```python
from build123d import *

# Parameters (mm, degrees)
SKETCH1_W             = 40
SKETCH1_H             = 84
SKETCH1_R             = 10.5
BOSS_EXTRUDE1_DEPTH   = 6
SKETCH2_W             = 40
SKETCH2_H             = 32
BOSS_EXTRUDE2_DEPTH   = 13
F_6_0MM_DOWEL_HOLE1_D = 6
M5_CLEARANCE_HOLE1_D  = 5.5
M4X0_7_TAPPED_HOLE1_D = 3.3
SKETCH12_R            = 17.5
CUT_EXTRUDE1_DEPTH    = 0.5
SKETCH13_R            = 17.5
CUT_EXTRUDE2_DEPTH    = 0.5
SKETCH14_W            = 33
SKETCH14_H            = 19
CUT_EXTRUDE3_DEPTH    = 5


with BuildPart() as part:
    # Sketch1 → Boss-Extrude1 (new body)
    with BuildSketch(Plane(origin=(0, 0, 0), x_dir=(1, 0, 0), z_dir=(0, 1, 0))):
        with Locations((0, -22)):
            Rectangle(SKETCH1_W, SKETCH1_H)
        Circle(SKETCH1_R, mode=Mode.SUBTRACT)
    extrude(amount=BOSS_EXTRUDE1_DEPTH)

    # Sketch2 → Boss-Extrude2 (add)
    with BuildSketch(Plane.XZ):
        with Locations((0, 48)):
            Rectangle(SKETCH2_W, SKETCH2_H)
    extrude(amount=BOSS_EXTRUDE2_DEPTH)

    # Ø6.0mm Dowel Hole1 (through all)
    with Locations(Plane(origin=(20, 0, 0), x_dir=(0, 0, -1), z_dir=(1, 0, 0))):
        with Locations((-57, -8), (-39, -8)):
            Hole(F_6_0MM_DOWEL_HOLE1_D / 2)

    # M5 Clearance Hole1 (through all)
    with Locations(Plane.ZY.offset(20)):
        with Locations((48, -8)):
            Hole(M5_CLEARANCE_HOLE1_D / 2)

    # M4x0.7 Tapped Hole1 (through all)
    with Locations(Plane(origin=(0, 0, 0), x_dir=(-1, 0, 0), z_dir=(0, -1, 0))):
        with Locations((16, 16), (-16, 16), (-16, -16), (16, -16)):
            Hole(M4X0_7_TAPPED_HOLE1_D / 2)

    # Sketch12 → Cut-Extrude1 (cut)
    with BuildSketch(Plane(origin=(0, 6, 0), x_dir=(1, 0, 0), z_dir=(0, 1, 0))):
        Circle(SKETCH12_R)
    extrude(amount=-CUT_EXTRUDE1_DEPTH, mode=Mode.SUBTRACT)

    # Sketch13 → Cut-Extrude2 (cut)
    with BuildSketch(Plane.XZ):
        Circle(SKETCH13_R)
    extrude(amount=-CUT_EXTRUDE2_DEPTH, mode=Mode.SUBTRACT)

    # Sketch14 → Cut-Extrude3 (cut)
    with BuildSketch(Plane(origin=(20, 0, 0), x_dir=(0, 0, -1), z_dir=(1, 0, 0))):
        with Locations((-47.5, -3.5)):
            Rectangle(SKETCH14_W, SKETCH14_H)
    extrude(amount=-CUT_EXTRUDE3_DEPTH, mode=Mode.SUBTRACT)


solid = part.part
```
Work out the finished part from the listing and answer in its coordinate system (mm). A direction names the side the tool comes from. Round coordinates to 2 decimals unless told otherwise and drop trailing zeros. Write each loop counter-clockwise with the first axis right and the second up, starting at its lowest first coordinate (ties: lowest second). Pieces come first, ordered by that corner, then holes. Notation, with made-up numbers: (79.25, -16.75) - (107.25, -16.75) arc R35 ccw to (107.25, 22.25) - close; hole circle Ø2 at (36, 27.5). An arc over 180 degrees is marked (long way). Return JSON: item names as keys, results as strings. Group by question number.
Q1. The part is cut by section A-A on x = 0. Write down the section's boundary in (y, z).
Q2. The part is cut by section C-C on y = -8. Write down the section's boundary in (x, z), then the cut area to 4 significant figures.
Q3. Each of these flat-tipped pins is pushed along its axis until it touches: pin 1 Ø4 at (x, z) = (16, 16) entering from -Y; pin 2 Ø1.5 at (x, y) = (3, -3.5) entering from -Z; pin 3 Ø2.5 at (x, y) = (16.5, 4.5) entering from +Z. Where does it stop, or does it pass through?
Q4. The mould has two halves that part along Y. Classify faces 1 (the cylindrical face through (-14.476, 3.042, -15.368)), 2 (the cylindrical face through (-2.255, -7.879, 50.747)), 3 (the flat face through (8, 0.5, -8)): released by +Y, released by -Y, zero draft, split by the parting line, or undercut.
Q5. For faces 4 (the flat face through (-5, 0, 17)), 5 (the flat face through (-3, -13, 48)), 6 (the flat face through (8, 5.5, 8)), 7 (the cylindrical face through (-13.887, 0.246, -10.648)), 8 (the flat face through (15, -3, 48)), determine the directions among +Z, -Z, +X, -X, +Y, -Y from which every point of the face is accessible in a straight line to the end or side of a thin tool.
Q6. The part is cut by section B-B on z = 0. Write down the section's boundary in (x, y), then the cut area to 3 significant figures.
Q7. Find the intervals of material crossed by L1, parallel to Z at x = 16, y = 1.75; L2, parallel to X at y = 2.55, z = 16; L3, parallel to Y at x = 8.5, z = 39, in increasing order.
Q8. The part is cut by section D-D on x = -16. Write down the section's boundary in (y, z).
Solved:
{
 "1": {"outline": "(-13, 32) - (0, 32) - (0, 17.5) - (0.5, 17.5) - (0.5, 10.5) - (5.5, 10.5) - (5.5, 17.5) - (6, 17.5) - (6, 64) - (-13, 64) - close; (0, -20) - (6, -20) - (6, -17.5) - (5.5, -17.5) - (5.5, -10.5) - (0.5, -10.5) - (0.5, -17.5) - (0, -17.5) - close; hole circle Ø6 at (-8, 39); hole circle Ø6 at (-8, 57); hole circle Ø5.5 at (-8, 48)"},
 "2": {"outline": "(-20, 32) - (15, 32) - (15, 36) - (-20, 36) - close; (-20, 42) - (15, 42) - (15, 45.25) - (-20, 45.25) - close; (-20, 50.75) - (15, 50.75) - (15, 54) - (-20, 54) - close; (-20, 60) - (15, 60) - (15, 64) - (-20, 64) - close", "area": "507.5 mm²"},
 "3": {"pin 1": "y = 0", "pin 2": "z = 32", "pin 3": "z = 31"},
 "4": {"face 1": "zero draft", "face 2": "undercut", "face 3": "released by -Y"},
 "5": {"face 4": "-Z, +X, -X, -Y", "face 5": "+Z, -Z, +X, -X, -Y", "face 6": "+Y", "face 7": "-Y", "face 8": "+Z, +X, +Y, -Y"},
 "6": {"outline": "(-20, 0) - (-17.5, 0) - (-17.5, 0.5) - (-10.5, 0.5) - (-10.5, 5.5) - (-17.5, 5.5) - (-17.5, 6) - (-20, 6) - close; (10.5, 0.5) - (17.5, 0.5) - (17.5, 0) - (20, 0) - (20, 6) - (17.5, 6) - (17.5, 5.5) - (10.5, 5.5) - close", "area": "100 mm²"},
 "7": {"L1": "-20 to -17.65, -14.35 to 14.35, 17.65 to 31", "L2": "-20 to -17.65, -14.35 to 14.35, 17.65 to 20", "L3": "-13 to -11, -5 to 6"},
 "8": {"outline": "(-13, 32) - (0, 32) - (0, 17.65) - (6, 17.65) - (6, 64) - (-13, 64) - close; (0, -20) - (6, -20) - (6, -17.65) - (0, -17.65) - close; (0, -14.35) - (6, -14.35) - (6, -7.09) - (5.5, -7.09) - (5.5, 7.09) - (6, 7.09) - (6, 14.35) - (0, 14.35) - (0, 7.09) - (0.5, 7.09) - (0.5, -7.09) - (0, -7.09) - close; hole circle Ø6 at (-8, 39); hole circle Ø6 at (-8, 57); hole circle Ø5.5 at (-8, 48)"}
}
